Verification items for the finished model (mm, model axes). Round coordinates to 2 decimals unless told otherwise and drop trailing zeros. Order: outer loops, then holes, each group sorted by start corner. A loop starts at its lowest first (then second) coordinate and runs counter-clockwise, first axis right, second up. Notation, with made-up numbers: (53, 79) -> (85, 79) arc R27 cw to (85, 114) -> close; hole circle Ø10 at (75, 86). An arc over 180 degrees is marked (long way). Return JSON: item names as keys, results as strings. Group by question number.
Item 1: Sectioned sample at B-B on y = -139. Record the cut outline in (x, z).
Item 2: Sectioned sample at A-A on x = -265. Record the cut outline in (y, z), plus the area to 3 significant figures.
Item 3: Depth check by flat-ended pin: pin 1 Ø1 at (x, z) = (-238, 3.5) entering from +Y; pin 2 Ø2.5 at (y, z) = (-60.5, 1.5) entering from +X; pin 3 Ø5 at (x, y) = (-36, -131) entering from +Z. Enter the tip coordinate at first touch or a pass-through.
Item 4: Scan lines: probe 1 along X at (y, z) = (-61.5, 0.5); probe 2 along Y at (x, z) = (-158.5, 1); probe 3 along Z at (x, y) = (-133, -130). Record each from-to range of solid material in increasing order. Write a range as from..to.
Item 5: Sectioned sample at C-C on x = -79.5. Record the cut outline in (y, z), plus the area to 3 significant figures.
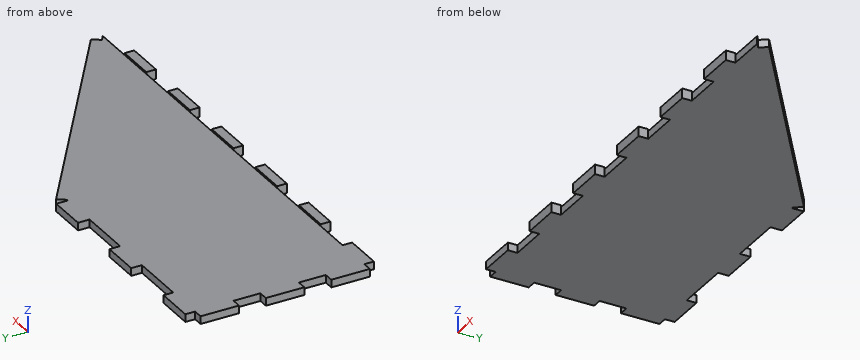
```python
from build123d import *

# Parameters (mm, degrees)
BOSS_EXTRUDE1_DEPTH = 5.08
SKETCH1_4_W         = 25.4
SKETCH1_4_H         = 6.35
BOSS_EXTRUDE2_DEPTH = 6.35
SKETCH1_5_W         = 25.4
SKETCH1_5_H         = 6.35
BOSS_EXTRUDE3_DEPTH = 6.35


with BuildPart() as part:
    # Sketch1 → Boss-Extrude1 (new body)
    with BuildSketch(Plane(origin=(-5.329574036, -16.20301374, 0), x_dir=(1, 0, 0), z_dir=(0, 0, 1))):
        Polygon((-288.637525151, -47.206627274), (-294.987525151, -47.206627274), (-294.987525151, -72.606627274), (-288.637525151, -72.606627274), (-288.637525151, -90.311124316), (-294.987525151, -90.311124316), (-294.987525151, -115.711124316), (-288.637525151, -115.711124316), (-288.637525151, -133.491124316), (-294.987525151, -133.491124316), (-294.987525151, -158.891124316), (-288.637525151, -158.891124316), (-288.637525151, -165.241124316), (-263.237525151, -165.241124316), (-263.237525151, -158.891124316), (16.162474849, -158.891124316), (12.459338773, -156.232709467), (16.162474849, -151.074290795), (-135.709389075, -42.048208602), (-139.412525151, -47.206627274), (-140.301525151, -47.206627274), (-140.301525151, -39.558279266), (-165.701525151, -39.558279266), (-165.701525151, -47.206627274), (-201.261525151, -47.206627274), (-201.261525151, -40.164648712), (-226.661525151, -40.164648712), (-226.661525151, -47.206627274), (-263.237525151, -47.206627274), (-263.237525151, -40.781124316), (-288.637525151, -40.781124316), align=None)
    extrude(amount=BOSS_EXTRUDE1_DEPTH)

    # Sketch1<4> → Boss-Extrude2 (add)
    with BuildSketch(Plane(origin=(-5.329574036, -16.20301374, 0), x_dir=(1, 0, 0), z_dir=(0, 0, 1))):
        with Locations((-225.137525151, -162.066124316)):
            Rectangle(SKETCH1_4_W, SKETCH1_4_H)
        with Locations((-174.337525151, -162.066124316)):
            Rectangle(SKETCH1_4_W, SKETCH1_4_H)
        with Locations((-123.537525151, -162.066124316)):
            Rectangle(SKETCH1_4_W, SKETCH1_4_H)
    extrude(amount=BOSS_EXTRUDE2_DEPTH)

    # Sketch1<5> → Boss-Extrude3 (add)
    with BuildSketch(Plane(origin=(-5.329574036, -16.20301374, 0), x_dir=(1, 0, 0), z_dir=(0, 0, 1))):
        with Locations((-72.737525151, -162.066124316)):
            Rectangle(SKETCH1_5_W, SKETCH1_5_H)
        with Locations((-21.937525151, -162.066124316)):
            Rectangle(SKETCH1_5_W, SKETCH1_5_H)
    extrude(amount=BOSS_EXTRUDE3_DEPTH)


solid = part.part
```
Recorded:
{
 "1": {"outline": "(-293.97, 0) -> (-28.56, 0) -> (-28.56, 5.08) -> (-293.97, 5.08) -> close"},
 "2": {"outline": "(-175.09, 0) -> (-63.41, 0) -> (-63.41, 5.08) -> (-175.09, 5.08) -> close", "area": "567 mm²"},
 "3": {"pin 1": "y = -63.41", "pin 2": "x = -136.17", "pin 3": "z = 5.08"},
 "4": {"probe 1": "-293.97..-268.57, -231.99..-206.59, -171.03..-145.63, -143.37..-136.51", "probe 2": "-175.09..-55.76", "probe 3": "0..5.08"},
 "5": {"outline": "(-181.44, 0) -> (-102.43, 0) -> (-102.43, 5.08) -> (-175.09, 5.08) -> (-175.09, 6.35) -> (-181.44, 6.35) -> close", "area": "409 mm²"}
}
